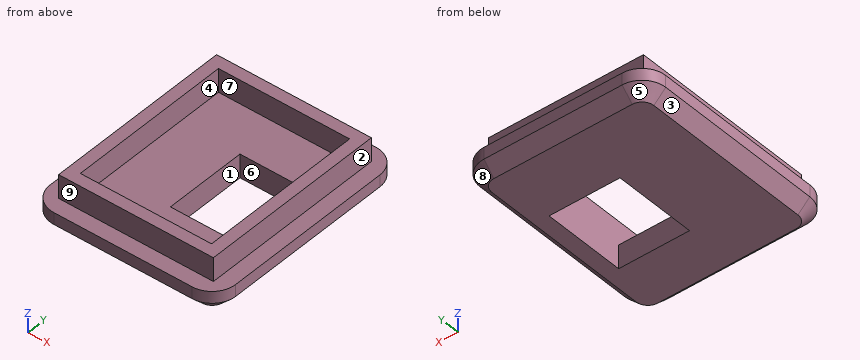
Autodesk Inventor part; units mm, degrees
ref_plane "YZ Plane" through (0, 0, 0) normal (1, 0, 0) x (0, 1, 0)
ref_plane "XZ Plane" through (0, 0, 0) normal (0, 1, 0) x (-1, 0, 0)
ref_plane "XY Plane" through (0, 0, 0) normal (0, 0, 1) x (1, 0, 0)
sketch "Sketch1" plane through (0, 0, 0) normal (0, 0, 1) x (1, 0, 0)
  point P0 (0, 0)
sketch "Sketch2" plane through (0, 0, 0) normal (0, 0, 1) x (1, 0, 0)
  point P0 (0, 0)
sketch "Sketch3" plane through (0, 0, 0) normal (0, 0, 1) x (1, 0, 0)
  line L0 (0, 0) -> (11.1, 0)
  line L1 (11.1, 0) -> (11.1, 13.9)
  line L2 (11.1, 13.9) -> (0, 13.9)
  line L3 (0, 13.9) -> (0, 0)
  line L4 (-1, -1) -> (12.1, -1)
  line L5 (12.1, -1) -> (12.1, 14.9)
  line L6 (12.1, 14.9) -> (-1, 14.9)
  line L7 (-1, 14.9) -> (-1, -1)
  dimension "d0" = 13.9
  dimension "d1" = 11.1
  dimension "d7" = 1
extrude "Extrusion1" add sketch "Sketch3" along normal blind 2
sketch "Sketch5" plane through (0, 0, 0) normal (0, 0, -1) x (-1, 0, 0)
  line L0 (-12.1, 14.9) -> (1, 14.9)
  line L1 (-12.1, -1) -> (-12.1, 14.9)
  line L2 (1, 14.9) -> (1, -1)
  line L3 (1, -1) -> (-12.1, -1)
  line L4 (2.3, 16.2) -> (-13.4, 16.2)
  line L5 (-13.4, 16.2) -> (-13.4, -2.3)
  line L6 (-13.4, -2.3) -> (2.3, -2.3)
  line L7 (2.3, -2.3) -> (2.3, 16.2)
  point P0 (0, 0)
  dimension "d8" = 1.3
extrude "Extrusion2" add sketch "Sketch5" along normal blind 2 contours L0 L2 L3 L1 | L7 L6 L5 L4
sketch "Sketch7" plane through (0, 0, 0) normal (0, 0, 1) x (1, 0, 0)
  line L0 (5.1, 3) -> (11.1, 3)
  line L1 (11.1, 3) -> (11.1, 10)
  line L2 (11.1, 10) -> (5.1, 10)
  line L3 (5.1, 10) -> (5.1, 3)
  line L4 (0, 0) -> (0, 13.9)
  line L5 (11.1, 0) -> (0, 0)
  line L6 (11.1, 13.9) -> (11.1, 0)
  dimension "d16" = 7
  dimension "d17" = 6
  dimension "d22" = 3
  dimension "d23" = 0
extrude "Extrusion4" cut sketch "Sketch7" against normal blind 2
fillet "Fillet1" radius 2 4 edges at (13.4, 16.2, -1) (-2.3, 16.2, -1) (13.4, -2.3, -1) (-2.3, -2.3, -1)
chamfer "Chamfer1" distance 1 angle 45 8 edges at (5.55, 16.2, -2) (12.8142, 15.6142, -2) (13.4, 6.95, -2) (12.8142, -1.7142, -2) (5.55, -2.3, -2) (-1.7142, -1.7142, -2) (-2.3, 6.95, -2) (-1.7142, 15.6142, -2)
properties part number "VL53L0X_cover_2"
Verification items for the finished model (mm, model axes). Face numbers are marked on the shaded views. A direction names the side the tool comes from. Coordinates: 2 decimals unless noted, no trailing zeros. Loops run counter-clockwise (first coordinate to the right, second up) from the corner with the lowest first, then second, coordinate; pieces in that order, holes last. Notation, with made-up numbers: (-29.75, 21) -> (-10.75, 21) arc R27 ccw to (-10.75, 59) -> close; hole circle Ø2 at (67.25, 0.25). An arc over 180 degrees is marked (long way). Answer as CSV lines item,"result".
1) Cross-section at C-C, the plane y = 4. Record the cut outline in (x, z), then the cut area to 3 significant figures.
Found:
outline,"(-2.3, -1) -> (-1.3, -2) -> (5.1, -2) -> (5.1, 0) -> (0, 0) -> (0, 2) -> (-1, 2) -> (-1, 0) -> (-2.3, 0) -> close; (11.1, -2) -> (12.4, -2) -> (13.4, -1) -> (13.4, 0) -> (12.1, 0) -> (12.1, 2) -> (11.1, 2) -> close"
area,"22.4 mm2"
2) Cross-section at A-A, the plane x = 7.5. Record the cut outline in (y, z), then the cut area to 3 significant figures.
Found:
outline,"(-2.3, -1) -> (-1.3, -2) -> (3, -2) -> (3, 0) -> (0, 0) -> (0, 2) -> (-1, 2) -> (-1, 0) -> (-2.3, 0) -> close; (10, -2) -> (15.2, -2) -> (16.2, -1) -> (16.2, 0) -> (14.9, 0) -> (14.9, 2) -> (13.9, 2) -> (13.9, 0) -> (10, 0) -> close"
area,"26.0 mm2"
3) Cross-section at D-D, the plane x = 1.5. Record the cut outline in (y, z), then the cut area to 3 significant figures.
Found:
outline,"(-2.3, -1) -> (-1.3, -2) -> (15.2, -2) -> (16.2, -1) -> (16.2, 0) -> (14.9, 0) -> (14.9, 2) -> (13.9, 2) -> (13.9, 0) -> (0, 0) -> (0, 2) -> (-1, 2) -> (-1, 0) -> (-2.3, 0) -> close"
area,"40.0 mm2"
4) Depth check by flat-ended pin: pin 1 (1.6 mm diameter, centred on y = 6, z = 1, fed in from +X); pin 2 (1.6 mm diameter, centred on x = 3.5, z = 1, fed in from +Y); pin 3 (1.6 mm diameter, centred on y = 9, z = 1, fed in from -X). Enter the tip coordinate at first touch or a pass-through.
Found:
pin 1,"stops at x = 12.1"
pin 2,"stops at y = 14.9"
pin 3,"stops at x = -1"
5) Cross-section at B-B, the plane z = 0.7. Record the cut outline in (x, y), then the cut area to 3 significant figures.
Found:
outline,"(-1, -1) -> (12.1, -1) -> (12.1, 14.9) -> (-1, 14.9) -> close; hole (0, 0) -> (11.1, 0) -> (11.1, 13.9) -> (0, 13.9) -> close"
area,"54.0 mm2"
6) Tool access check on the marked faces 5, 6, 7, 8 and 9. Record the directions out of +Z, -Z, +X, -X, +Y, -Y that give a thin tool (end or side, any length) a straight path to the whole face; none if there is none.
Found:
face 5,"-Z, -X, +Y"
face 6,"+Z, -Z"
face 7,"+Z"
face 8,"-Z, +X, +Y"
face 9,"+Z, +X, -X, -Y"
7) Thickness scan on L1, parallel to Y at x = 3, z = 1.35; L2, parallel to X at y = 3, z = 1.05; L3, parallel to Y at x = 9.5, z = -0.35. Record the ranges inside material, lowest first. Write a range as from..to.
Found:
L1,"y = -1..0, 13.9..14.9"
L2,"x = -1..0, 11.1..12.1"
L3,"y = -2.3..3, 10..16.2"
8) Release check for a two-part mould opening along X. For the marked faces 1, 2, 3 and 4 record: +X half, -X half, draft (parallel to the pull), parting line (faces both ways), or undercut.
Found:
face 1,"undercut"
face 2,"+X half"
face 3,"-X half"
face 4,"undercut"
